```python
from build123d import *

# Parameters (mm, degrees)
F0_W     = 530
F0_H     = 345
F0_R     = 2.5
F0_W_2   = 2
F0_H_2   = 10
F0_W_3   = 470
F0_H_3   = 265
F1_DEPTH = 3
F2_W     = 470
F2_H     = 265
F2_R     = 2.5
F2_W_2   = 2
F2_H_2   = 10
F3_DEPTH = 1
F4_W     = 390
F4_H     = 295
F4_H_2   = 245
F5_DEPTH = 30


with BuildPart() as f1:
    # F0 (on Front) → F1 (new body)
    with BuildSketch(Plane.XZ):
        Rectangle(F0_W, F0_H)
        with Locations((-212.5, -145)):
            Circle(F0_R, mode=Mode.SUBTRACT)
        with Locations((0, -147.5)):
            Rectangle(F0_W_2, F0_H_2, mode=Mode.SUBTRACT)
        with Locations((0, 10)):
            Rectangle(F0_W_3, F0_H_3, mode=Mode.SUBTRACT)
        with Locations((0, 10)):
            Rectangle(F0_W_3, F0_H_3)
        with Locations((0, -147.5)):
            Rectangle(F0_W_2, F0_H_2)
        with Locations((-212.5, -145)):
            Circle(F0_R)
    extrude(amount=F1_DEPTH)

    # F2 (on face) → F3 (cut)
    with BuildSketch(Plane.XZ.offset(3)):
        with Locations((0, 10)):
            Rectangle(F2_W, F2_H)
        with Locations((-212.5, -145)):
            Circle(F2_R)
        with Locations((0, -147.5)):
            Rectangle(F2_W_2, F2_H_2)
    extrude(amount=-F3_DEPTH, mode=Mode.SUBTRACT)

    # F4 (on face) → F5 (join)
    with BuildSketch(Plane.XZ):
        with Locations((0, -25)):
            Rectangle(F4_W, F4_H)
        Rectangle(F4_W, F4_H_2)
    extrude(amount=-F5_DEPTH)


solid = f1.part
```
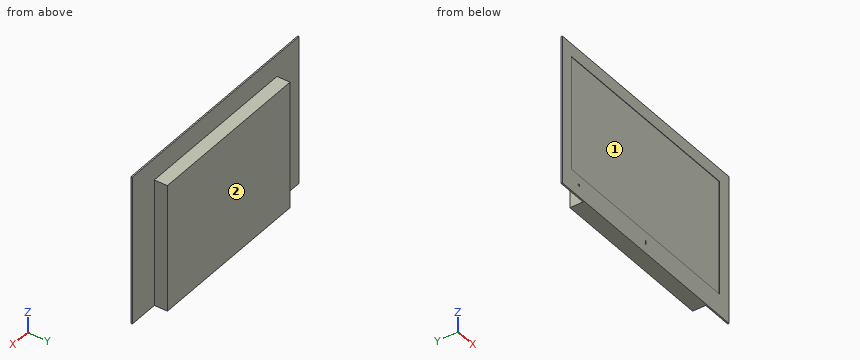
CAD build for the part. Positions are in the model's coordinates, mm. Face numbers are marked on the shaded views. Round coordinates to 2 decimals unless told otherwise and drop trailing zeros. Loops run counter-clockwise (first coordinate to the right, second up) from the corner with the lowest first, then second, coordinate; pieces in that order, holes last. Notation, with made-up numbers: M -27,41.5 L 26,41.5 A9 ccw 26,47.5 Z; hole C 7.25,70 d8. An arc over 180 degrees is marked long. Use a Markdown table: item, result. Add a question column.
(1) Cut at B-B (z = 1.5). Give the cut face in (x, y), and give its area (3 significant figures).
(2) Cut at A-A (x = -25.5). Give the cut face in (y, z).
(3) Flat gauge pins, fed straight in: pin 1 (8 mm diameter, centred on x = -17, z = 96.5, fed in from -Y); pin 2 (10 mm diameter, centred on y = 14, z = -121.5, fed in from -X); pin 3 (15 mm diameter, centred on x = 25.5, y = 10, fed in from +Z). Where does each tip first touch, or does it go through?
(4) Drill centre lines: line 1 (Z direction, x = -212.5, y = -2.5); line 2 (X direction, y = -2.25, z = -145); line 3 (X direction, y = 2, z = -123.5). Where is each one in solid material? Low to high.
(5) Cut at C-C (y = 21.5). Give the cut face in (x, z), and give its area (3 significant figures).
(6) Pull direction X, two halves, no side cores. Call the marked faces 1 and 2: +X half, -X half, draft (parallel to the pull), parting line (faces both ways), or undercut.
Geometry says:
| question | item | result |
|---|---|---|
| 1 | outline | M -265,-3 L -235,-3 L -235,-2 L 235,-2 L 235,-3 L 265,-3 L 265,0 L 195,0 L 195,30 L -195,30 L -195,0 L -265,0 Z |
| 1 | area | 12,800 mm² |
| 2 | outline | M -3,-172.5 L 30,-172.5 L 30,122.5 L 0,122.5 L 0,172.5 L -3,172.5 L -3,142.5 L -2,142.5 L -2,-122.5 L -3,-122.5 Z |
| 3 | pin 1 | stops at y = -2 |
| 3 | pin 2 | stops at x = -195 |
| 3 | pin 3 | stops at z = 122.5 |
| 4 | line 1 | z = -172.5 to -147.5, -142.5 to -122.5, 142.5 to 172.5 |
| 4 | line 2 | x = -265 to -215, -210 to -1, 1 to 265 |
| 4 | line 3 | x = -195 to 195 |
| 5 | outline | M -195,-172.5 L 195,-172.5 L 195,122.5 L -195,122.5 Z |
| 5 | area | 115,000 mm² |
| 6 | face 1 | undercut |
| 6 | face 2 | draft |
